from build123d import *

# Parameters (mm, degrees)
EXTRUDE_1_DEPTH = 100


with BuildPart() as part:
    # 草图1 → 凸台-拉伸1 (new body)
    with BuildSketch(Plane.XY):
        with BuildLine():
            Line((-4.329808423, 24.195670518), (-24.229808423, 24.195670518))
            ThreePointArc((-24.229808423, 24.195670518), (-24.936915205, 23.902777299), (-25.229808423, 23.195670518))
            Line((-25.229808423, 23.195670518), (-25.229808423, 3.295670518))
            Line((-25.229808423, 3.295670518), (-23.229808423, 3.295670518))
            Line((-23.229808423, 3.295670518), (-23.229808423, 6.645670518))
            Line((-23.229808423, 6.645670518), (-13.229808423, 6.645670518))
            Line((-13.229808423, 6.645670518), (-13.229808423, 3.295670518))
            Line((-13.229808423, 3.295670518), (-9.229808423, 3.295670518))
            Line((-9.229808423, 3.295670518), (-9.229808423, -4.904329482))
            Line((-9.229808423, -4.904329482), (-13.229808423, -4.904329482))
            Line((-13.229808423, -4.904329482), (-13.229808423, -8.254329482))
            Line((-13.229808423, -8.254329482), (-23.229808423, -8.254329482))
            Line((-23.229808423, -8.254329482), (-23.229808423, -4.904329482))
            Line((-23.229808423, -4.904329482), (-25.229808423, -4.904329482))
            Line((-25.229808423, -4.904329482), (-25.229808423, -24.804329482))
            ThreePointArc((-25.229808423, -24.804329482), (-24.936915205, -25.511436263), (-24.229808423, -25.804329482))
            Line((-24.229808423, -25.804329482), (-4.329808423, -25.804329482))
            Line((-4.329808423, -25.804329482), (-4.329808423, -23.804329482))
            Line((-4.329808423, -23.804329482), (-7.679808423, -23.804329482))
            Line((-7.679808423, -23.804329482), (-7.679808423, -13.804329482))
            Line((-7.679808423, -13.804329482), (-4.329808423, -13.804329482))
            Line((-4.329808423, -13.804329482), (-4.329808423, -9.804329482))
            Line((-4.329808423, -9.804329482), (3.870191577, -9.804329482))
            Line((3.870191577, -9.804329482), (3.870191577, -13.804329482))
            Line((3.870191577, -13.804329482), (7.220191577, -13.804329482))
            Line((7.220191577, -13.804329482), (7.220191577, -23.804329482))
            Line((7.220191577, -23.804329482), (3.870191577, -23.804329482))
            Line((3.870191577, -23.804329482), (3.870191577, -25.804329482))
            Line((3.870191577, -25.804329482), (23.770191577, -25.804329482))
            ThreePointArc((23.770191577, -25.804329482), (24.477298358, -25.511436263), (24.770191577, -24.804329482))
            Line((24.770191577, -24.804329482), (24.770191577, -4.904329482))
            Line((24.770191577, -4.904329482), (22.770191577, -4.904329482))
            Line((22.770191577, -4.904329482), (22.770191577, -8.254329482))
            Line((22.770191577, -8.254329482), (12.770191577, -8.254329482))
            Line((12.770191577, -8.254329482), (12.770191577, -4.904329482))
            Line((12.770191577, -4.904329482), (8.770191577, -4.904329482))
            Line((8.770191577, -4.904329482), (8.770191577, 3.295670518))
            Line((8.770191577, 3.295670518), (12.770191577, 3.295670518))
            Line((12.770191577, 3.295670518), (12.770191577, 6.645670518))
            Line((12.770191577, 6.645670518), (22.770191577, 6.645670518))
            Line((22.770191577, 6.645670518), (22.770191577, 3.295670518))
            Line((22.770191577, 3.295670518), (24.770191577, 3.295670518))
            Line((24.770191577, 3.295670518), (24.770191577, 23.195670518))
            ThreePointArc((24.770191577, 23.195670518), (24.477298358, 23.902777299), (23.770191577, 24.195670518))
            Line((23.770191577, 24.195670518), (3.870191577, 24.195670518))
            Line((3.870191577, 24.195670518), (3.870191577, 22.195670518))
            Line((3.870191577, 22.195670518), (7.220191577, 22.195670518))
            Line((7.220191577, 22.195670518), (7.220191577, 12.195670518))
            Line((7.220191577, 12.195670518), (3.870191577, 12.195670518))
            Line((3.870191577, 12.195670518), (3.870191577, 8.195670518))
            Line((3.870191577, 8.195670518), (-4.329808423, 8.195670518))
            Line((-4.329808423, 8.195670518), (-4.329808423, 12.195670518))
            Line((-4.329808423, 12.195670518), (-7.679808423, 12.195670518))
            Line((-7.679808423, 12.195670518), (-7.679808423, 22.195670518))
            Line((-7.679808423, 22.195670518), (-4.329808423, 22.195670518))
            Line((-4.329808423, 22.195670518), (-4.329808423, 24.195670518))
        make_face()
        with BuildLine():
            Line((-23.229808423, 8.645670518), (-9.979808423, 8.645670518))
            ThreePointArc((-9.979808423, 8.645670518), (-9.767676389, 8.733538484), (-9.679808423, 8.945670518))
            Line((-9.679808423, 8.945670518), (-9.679808423, 21.895670518))
            ThreePointArc((-9.679808423, 21.895670518), (-9.767676389, 22.107802553), (-9.979808423, 22.195670518))
            Line((-9.979808423, 22.195670518), (-22.929808423, 22.195670518))
            ThreePointArc((-22.929808423, 22.195670518), (-23.141940458, 22.107802553), (-23.229808423, 21.895670518))
            Line((-23.229808423, 21.895670518), (-23.229808423, 8.645670518))
        make_face(mode=Mode.SUBTRACT)
        with BuildLine():
            Line((22.770191577, 8.645670518), (9.520191577, 8.645670518))
            ThreePointArc((9.520191577, 8.645670518), (9.308059542, 8.733538484), (9.220191577, 8.945670518))
            Line((9.220191577, 8.945670518), (9.220191577, 21.895670518))
            ThreePointArc((9.220191577, 21.895670518), (9.308059542, 22.107802553), (9.520191577, 22.195670518))
            Line((9.520191577, 22.195670518), (22.470191577, 22.195670518))
            ThreePointArc((22.470191577, 22.195670518), (22.682323611, 22.107802553), (22.770191577, 21.895670518))
            Line((22.770191577, 21.895670518), (22.770191577, 8.645670518))
        make_face(mode=Mode.SUBTRACT)
        with BuildLine():
            Line((-23.229808423, -10.254329482), (-9.979808423, -10.254329482))
            ThreePointArc((-9.979808423, -10.254329482), (-9.767676389, -10.342197447), (-9.679808423, -10.554329482))
            Line((-9.679808423, -10.554329482), (-9.679808423, -23.504329482))
            ThreePointArc((-9.679808423, -23.504329482), (-9.767676389, -23.716461516), (-9.979808423, -23.804329482))
            Line((-9.979808423, -23.804329482), (-22.929808423, -23.804329482))
            ThreePointArc((-22.929808423, -23.804329482), (-23.141940458, -23.716461516), (-23.229808423, -23.504329482))
            Line((-23.229808423, -23.504329482), (-23.229808423, -10.254329482))
        make_face(mode=Mode.SUBTRACT)
        with BuildLine():
            Line((22.770191577, -10.254329482), (9.520191577, -10.254329482))
            ThreePointArc((9.520191577, -10.254329482), (9.308059542, -10.342197447), (9.220191577, -10.554329482))
            Line((9.220191577, -10.554329482), (9.220191577, -23.504329482))
            ThreePointArc((9.220191577, -23.504329482), (9.308059542, -23.716461516), (9.520191577, -23.804329482))
            Line((9.520191577, -23.804329482), (22.470191577, -23.804329482))
            ThreePointArc((22.470191577, -23.804329482), (22.682323611, -23.716461516), (22.770191577, -23.504329482))
            Line((22.770191577, -23.504329482), (22.770191577, -10.254329482))
        make_face(mode=Mode.SUBTRACT)
        with BuildLine():
            ThreePointArc((2.451084423, 2.933693197), (-0.229808423, 3.795670518), (-2.91070127, 2.933693197))
            ThreePointArc((-2.91070127, 2.933693197), (-4.012829703, 2.978691798), (-3.967831102, 1.876563365))
            ThreePointArc((-3.967831102, 1.876563365), (-4.829808423, -0.804329482), (-3.967831102, -3.485222328))
            ThreePointArc((-3.967831102, -3.485222328), (-4.012829703, -4.587350761), (-2.91070127, -4.54235216))
            ThreePointArc((-2.91070127, -4.54235216), (-0.229808423, -5.404329482), (2.451084423, -4.54235216))
            ThreePointArc((2.451084423, -4.54235216), (3.553212856, -4.587350761), (3.508214255, -3.485222328))
            ThreePointArc((3.508214255, -3.485222328), (4.370191577, -0.804329482), (3.508214255, 1.876563365))
            ThreePointArc((3.508214255, 1.876563365), (3.553212856, 2.978691798), (2.451084423, 2.933693197))
        make_face(mode=Mode.SUBTRACT)
    extrude(amount=EXTRUDE_1_DEPTH)


solid = part.part
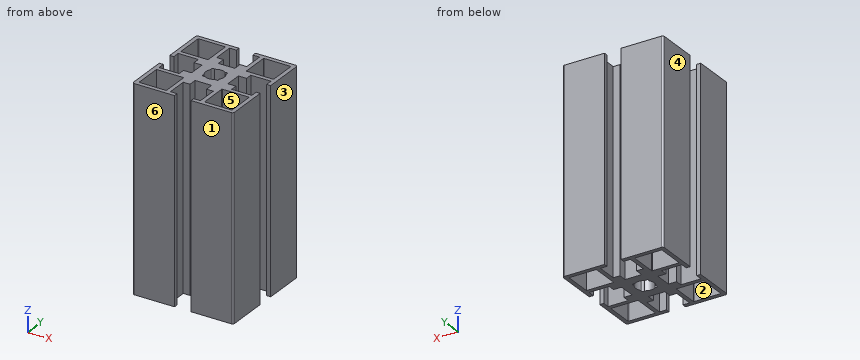
Read the model definition and answer for the solid it produces. Units are mm, in the model's axes. Face numbers are marked on the shaded views. A direction names the side the tool comes from. Round coordinates to 2 decimals unless told otherwise and drop trailing zeros. Write each loop counter-clockwise with the first axis right and the second up, starting at its lowest first coordinate (ties: lowest second). Pieces come first, ordered by that corner, then holes. Notation, with made-up numbers: (20, 48.5) - (62, 48.5) arc R31 ccw to (62, 83.5) - close; hole circle Ø6 at (87.5, 72.25). An arc over 180 degrees is marked (long way). One line per question, with ' | ' between items. Start each with the question number.
1. Section C-C (z = 13) is taken. Give the number of separate pieces and of enclosed holes in the cut face, and give its area (3 significant figures).
2. Section A-A (y = -20) is taken. Determine the outline of the cut face in (x, z).
3. For the marked faces 5 and 6, determine the directions among +Z, -Z, +X, -X, +Y, -Y from which every point of the face is accessible in a straight line to the end or side of a thin tool.
4. For a pull along X with two mould halves and no side action, classify the marked faces 1, 2, 3 and 4 as +X half, -X half, draft (parallel to the pull), parting line (faces both ways), or undercut.
5. Find the intervals of material crossed by probe 1 along Y at (x, z) = (-18, 29); probe 2 along X at (y, z) = (20.5, 61); probe 3 along X at (y, z) = (12, 45), in increasing order. Write a range as [from, to].
6. Section D-D (x = 0.5) is taken. Determine the outline of the cut face in (y, z), and give its area (3 significant figures).
7. Section B-B (x = -6.5) is taken. Determine the outline of the cut face in (y, z), and give its area (3 significant figures).
Filled in:
1) separate pieces: 1 | enclosed holes: 5 | area: 902 mm²
2) outline: (-25.23, 0) - (-23.23, 0) - (-23.23, 100) - (-25.23, 100) - close; (-9.68, 0) - (-7.68, 0) - (-7.68, 100) - (-9.68, 100) - close; (7.22, 0) - (9.22, 0) - (9.22, 100) - (7.22, 100) - close; (22.77, 0) - (24.77, 0) - (24.77, 100) - (22.77, 100) - close
3) face 5: +Z, -Z | face 6: +Z, -Z, +X, -X, -Y
4) face 1: draft | face 2: undercut | face 3: +X half | face 4: -X half
5) probe 1: [-25.8, -23.8], [-10.25, -8.25], [6.65, 8.65], [22.2, 24.2] | probe 2: [-25.23, -23.23], [-9.68, -7.68], [7.22, 9.22], [22.77, 24.77] | probe 3: [-25.23, -23.23], [-9.68, -4.33], [3.87, 9.22], [22.77, 24.77]
6) outline: (-9.8, 0) - (-5.35, 0) - (-5.35, 100) - (-9.8, 100) - close; (3.74, 0) - (8.2, 0) - (8.2, 100) - (3.74, 100) - close | area: 892 mm²
7) outline: (-25.8, 0) - (-23.8, 0) - (-23.8, 100) - (-25.8, 100) - close; (-13.8, 0) - (12.2, 0) - (12.2, 100) - (-13.8, 100) - close; (22.2, 0) - (24.2, 0) - (24.2, 100) - (22.2, 100) - close | area: 3,000 mm²
